Verification items for the finished model (mm, model axes). Face numbers are marked on the shaded views. A direction names the side the tool comes from. Give positions to 0.01 mm unless a question says otherwise; leave off trailing zeros. Order: outer loops, then holes, each group sorted by start corner. A loop starts at its lowest first (then second) coordinate and runs counter-clockwise, first axis right, second up.
(1) Sectioned sample at D-D on y = 15. Record the cut outline in (x, z), plus the area to 3 significant figures.
(2) Sectioned sample at B-B on z = 11. Record the cut outline in (x, y).
(3) Access from +Z, -Z, +X, -X, +Y, -Y to the whole of each face (thin tool, end or side, straight path). Record for the marked faces 5 and 6.
(4) Sectioned sample at C-C on y = 0. Record the cut outline in (x, z), plus the area to 3 significant figures.
(5) Gauge pin test, flat ends, axial feed: pin 1 (10 mm diameter, centred on y = -1, z = 10, fed in from +X); pin 2 (3 mm diameter, centred on y = 3.5, z = 6.5, fed in from -X); pin 3 (4 mm diameter, centred on y = 16.5, z = 9, fed in from -X). Record the tip position at first contact, or that the pin passes through.
(6) Mould release check, pull along X, two halves, no side actions. Record for the marked faces 1, 2, 3 and 4: pulls with the +X half, pulls with the -X half, needs draft (parallel to the pull), parting line crosses it, or undercut.
(7) Scan lines: L1, parallel to Y at x = 25, z = -2.7; L2, parallel to Z at x = 11.35, y = 15; L3, parallel to Z at x = 31.5, y = 2. Record each from-to range of solid material in increasing order.
(8) Sectioned sample at A-A on x = 25. Record the cut outline in (y, z).
Autodesk Fusion 360 part; units mm, degrees
sketch "スケッチ1" plane through (0, 0, 0) normal (0, 0, 1) x (1, 0, 0)
  circle A0 centre (0, 0) radius 2.25
  circle A1 centre (0, 0) radius 7
  line L0 (-2.0936, 6.6796) -> (8.5, 10)
  line L1 (8.5, 10) -> (35, 10)
  line L2 (35, 10) -> (35, -10)
  line L3 (35, -10) -> (8.5, -10)
  line L4 (8.5, -10) -> (-2.0936, -6.6796)
  circle A2 centre (25, 0) radius 2.7
  line L5 (25, 2.7) -> (35, 2.7)
  line L6 (25, -2.7) -> (35, -2.7)
  line L7 (35, 10) -> (10, 10)
  line L8 (10, 10) -> (10, 20)
  line L9 (10, 20) -> (35, 20)
  line L10 (35, 20) -> (35, 10)
  line L11 (10, 20) -> (15, 20)
  line L12 (15, 20) -> (15, 10)
  line L13 (15, 10) -> (10, 10)
  line L14 (10, 10) -> (10, 20)
  line L15 (10, -10) -> (10, 10)
  dimension "d1" = 14
  dimension "d2" = 4.5
  dimension "d3" = 35
  dimension "d4" = 10
  dimension "d5" = 10
  dimension "d6" = 26.5
  dimension "d7" = 26.5
  dimension "d8" = 5.4
  dimension "d9" = 10
  dimension "d36" = 10
  dimension "d37" = 25
  dimension "d38" = 5
  dimension "d47" = 25
extrude "押し出し1" add sketch "スケッチ1" against normal blind 5 contours A1 | A1 L0 L1 L3 L4 L15 | L1 L2 L3 A2 L5 L6 L7 L13 L15 | L2 A2 L5 L6
sketch "スケッチ2" plane through (0, 0, 0) normal (0, 0, 1) x (1, 0, 0)
  line L0 (8.5, 10) -> (35, 10)
  line L1 (35, -10) -> (8.5, -10)
  line L2 (15, 10) -> (15, -10)
  line L3 (8.5, 10) -> (8.5, -10)
  line L4 (10, 10) -> (10, -10)
  line L5 (8.5, 5) -> (10, 5)
  line L6 (8.5, -5) -> (10, -5)
  dimension "d12" = 1.5
  dimension "d13" = 5
  dimension "d14" = 5
  dimension "d15" = 5
extrude "押し出し2" add sketch "スケッチ2" along normal blind 20 contours L0 L1 L2 L4
extrude "Extrude6" add sketch "スケッチ1" along normal up to surface (20 mm away) contours A1 | A1 L0 L1 L3 L4 L15
fillet "フィレット1" radius 1 2 edges at (15, -10, 10) (35, -10, -2.5)
extrude "Extrude3" add sketch "スケッチ1" against normal blind 5 contours L1 L7 L8 L9 L11 L12 L13 L14 | L1 L7 L9 L10 L12
extrude "Extrude4" add sketch "スケッチ1" along normal up to surface (20 mm away) contours L1 L7 L8 L9 L11 L12 L13 L14
sketch "Sketch3" plane through (10, 0, 0) normal (-1, 0, 0) x (0, -1, 0)
  line L0 (-20, 20) -> (-20, -5)
  line L1 (-20, -5) -> (-10, -5)
  line L2 (-10, -5) -> (-10, 20)
  line L3 (-10, 20) -> (-20, 20)
  line L4 (-10, 0) -> (-20, 0) construction
  line L5 (-15, 0) -> (-15, 20) construction
  line L6 (-20, 0) -> (-20, 20) construction
  line L7 (-20, 10) -> (-10, 10) construction
  circle A0 centre (-15, 10) radius 2.7
  dimension "d43" = 5.4
extrude "Extrude5" cut sketch "Sketch3" against normal blind 5 contours A0
fillet "Fillet7" radius 1 8 edges at (15, 20, 10) (10, 20, 7.5) (35, 0.5, 0) (35, 15, 0) (34.7071, -9.7071, 0) (24, -10, 0) (25, 20, 0) (35, 20, -2.5)
fillet "Fillet9" radius 1 1 edges at (10, 10, 7.5)
equation "d3 = 29 mm + 6 mm"
equation "d6 = 20.5 mm + 6 mm"
equation "d7 = 20.5 mm + 6 mm"
equation "d9 = 4 mm + 6 mm"
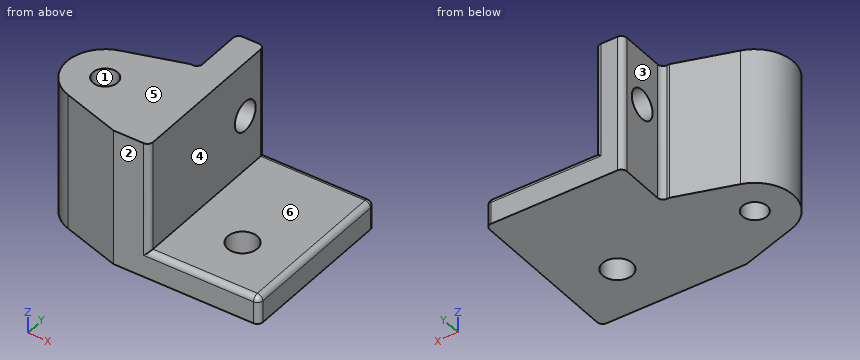
Ans:
1. outline: (10, -5) - (35, -5) - (35, -1) arc R1 ccw to (34, 0) - (15, 0) - (15, 7.3) - (10, 7.3) - close; (10, 12.7) - (15, 12.7) - (15, 20) - (10, 20) - close
1. area: 198 mm2
2. outline: (-2.09, -6.68) - (8.5, -10) - (14, -10) arc R1 ccw to (15, -9) - (15, 12.49) - (10, 12.49) - (10, 11) arc R1 cw to (9, 10) - (8.5, 10) - (-2.09, 6.68) arc R7 ccw to start; (10, 17.51) - (15, 17.51) - (15, 19) arc R1 ccw to (14, 20) - (11, 20) arc R1 ccw to (10, 19) - close; hole circle Ø4.5 at (0, 0)
3. face 5: +Z, +X, -X, +Y, -Y
3. face 6: +Z, +X, +Y, -Y
4. outline: (-7, -5) - (-2.25, -5) - (-2.25, 20) - (-7, 20) - close; (2.25, -5) - (22.3, -5) - (22.3, 0) - (15, 0) - (15, 20) - (2.25, 20) - close; (27.7, -5) - (35, -5) - (35, -1) arc R1 ccw to (34, 0) - (27.7, 0) - close
4. area: 510 mm2
5. pin 1: stops at x = 15
5. pin 2: stops at x = -6.71
5. pin 3: stops at x = 10
6. face 1: undercut
6. face 2: needs draft
6. face 3: pulls with the -X half
6. face 4: pulls with the +X half
7. L1: y = -10 to -2.7, 2.7 to 20
7. L2: z = -5 to 7.3, 12.7 to 20
7. L3: z = -5 to 0
8. outline: (-10, -5) - (-2.7, -5) - (-2.7, 0) - (-9, 0) arc R1 ccw to (-10, -1) - close; (2.7, -5) - (20, -5) - (20, -1) arc R1 ccw to (19, 0) - (2.7, 0) - close
